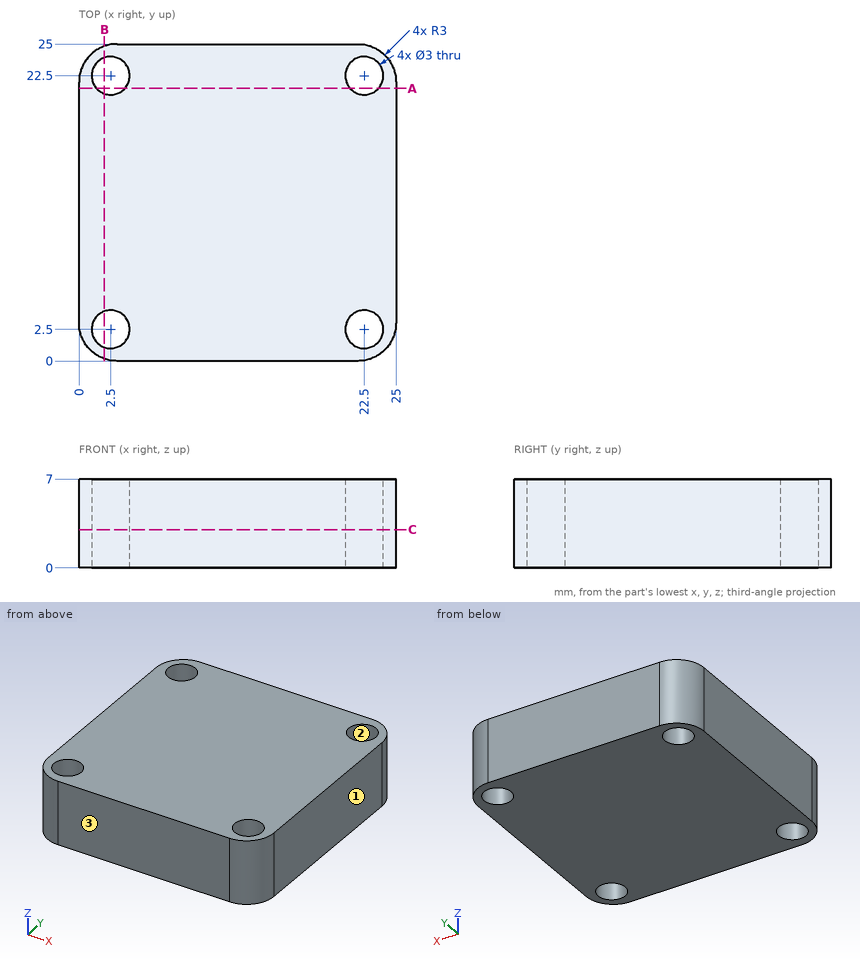
Source: three-view drawing plus pictorial views. Frame: mm from the lowest corner of the part. Round coordinates to 2 decimals unless told otherwise and drop trailing zeros. Loops run counter-clockwise (first coordinate to the right, second up) from the corner with the lowest first, then second, coordinate; pieces in that order, holes last. Notation, with made-up numbers: M -31,62 L 25,62 A29 cw 25,85 Z; hole C -22.5,-34.5 d11. An arc over 180 degrees is marked long. Answer as CSV lines item,"result".
Q1. Line query: line 1 along Y through (x, z) = (2.5, 2); line 2 along Y through (x, z) = (22, 5.25); line 3 along X through (y, z) = (1.5, 6.75). Output: solid intervals per line, ascending.
Verdict:
line 1,"y = 0.04 to 1, 4 to 21, 24 to 24.96"
line 2,"y = 0 to 1.09, 3.91 to 21.09, 23.91 to 25"
line 3,"x = 0.4 to 1.38, 3.62 to 21.38, 23.62 to 24.6"
Q2. Cut plane A-A (y = 21.5). Return the cut outline in (x, z), plus the area to 3 significant figures.
Verdict:
outline,"M 0,0 L 1.38,0 L 1.38,7 L 0,7 Z; M 3.62,0 L 21.38,0 L 21.38,7 L 3.62,7 Z; M 23.62,0 L 25,0 L 25,7 L 23.62,7 Z"
area,"144 mm^2"
Q3. Pull-direction query (X, two-part tool) for the marked faces 1, 2 and 3; classes: +X half, -X half, draft (parallel to the pull), parting line (faces both ways), or undercut.
Verdict:
face 1,"+X half"
face 2,"undercut"
face 3,"draft"
Q4. Cut plane C-C (z = 3). Return the cut outline in (x, y).
Verdict:
outline,"M 0,3 A3 ccw 3,0 L 22,0 A3 ccw 25,3 L 25,22 A3 ccw 22,25 L 3,25 A3 ccw 0,22 Z; hole C 2.5,2.5 d3; hole C 2.5,22.5 d3; hole C 22.5,2.5 d3; hole C 22.5,22.5 d3"
Q5. Cut plane B-B (x = 2). Return the cut outline in (y, z).
Verdict:
outline,"M 0.17,0 L 1.09,0 L 1.09,7 L 0.17,7 Z; M 3.91,0 L 21.09,0 L 21.09,7 L 3.91,7 Z; M 23.91,0 L 24.83,0 L 24.83,7 L 23.91,7 Z"
